```python
from build123d import *

# Parameters (mm, degrees)
F0_W      = 72
F0_H      = 30
F1_DEPTH  = 4
F3_DEPTH  = 5
F4_R      = 3.75
F5_DEPTH  = 9.001
F8_DEPTH  = 15
F10_DEPTH = 25
F12_DEPTH = 3
F13_R     = 1.65
F14_DEPTH = 3


with BuildPart() as f1:
    # F0 (on Top) → F1 (new body)
    with BuildSketch(Plane.XY):
        with BuildLine():
            ThreePointArc((37.445899, 13.116578), (35.981432, 16.652112), (32.445899, 18.116578))
            Line((32.445899, 18.116578), (-32.554101, 18.116578))
            ThreePointArc((-32.554101, 18.116578), (-36.089635, 16.652112), (-37.554101, 13.116578))
            Line((-37.554101, 13.116578), (-37.554101, -9.883422))
            Line((-37.554101, -9.883422), (-37.554101, -14.883422))
            Line((-37.554101, -14.883422), (-32.554101, -14.883422))
            Line((-32.554101, -14.883422), (32.445899, -14.883422))
            ThreePointArc((32.445899, -14.883422), (35.981432, -13.418956), (37.445899, -9.883422))
            Line((37.445899, -9.883422), (37.445899, 13.116578))
        make_face()
        with Locations((-0.054101, 1.616578)):
            Rectangle(F0_W, F0_H, mode=Mode.SUBTRACT)
    extrude(amount=F1_DEPTH)

    # F2 (on face) → F3 (join)
    with BuildSketch(Plane(origin=(0, 0, 0), x_dir=(1, 0, 0), z_dir=(0, 0, -1))):
        with BuildLine():
            Line((32.445899, 14.883422), (-37.554101, 14.883422))
            Line((-37.554101, 14.883422), (-37.554101, -13.116578))
            ThreePointArc((-37.554101, -13.116578), (-36.089635, -16.652112), (-32.554101, -18.116578))
            Line((-32.554101, -18.116578), (32.445899, -18.116578))
            ThreePointArc((32.445899, -18.116578), (35.981432, -16.652112), (37.445899, -13.116578))
            Line((37.445899, -13.116578), (37.445899, 9.883422))
            ThreePointArc((37.445899, 9.883422), (35.981432, 13.418956), (32.445899, 14.883422))
        make_face()
    extrude(amount=F3_DEPTH)

    # F4 (on face) → F5 (cut, through all)
    with BuildSketch(Plane(origin=(0, 0, -5), x_dir=(1, 0, 0), z_dir=(0, 0, -1))):
        with Locations((8, -1.616578)):
            Circle(F4_R)
    extrude(amount=-F5_DEPTH, mode=Mode.SUBTRACT)

    # F7 (on face) → F8 (join)
    with BuildSketch(Plane(origin=(0, 0, -5), x_dir=(1, 0, 0), z_dir=(0, 0, -1))):
        with BuildLine():
            ThreePointArc((2.992242, -13.613343), (-5, -1.616578), (2.992242, 10.380186))
            Line((2.992242, 10.380186), (2.992242, 11.45715))
            ThreePointArc((2.992242, 11.45715), (-6, -1.616578), (2.992242, -14.690306))
            Line((2.992242, -14.690306), (2.992242, -13.613343))
        make_face()
        with BuildLine():
            ThreePointArc((13.007758, -14.690306), (22, -1.616578), (13.007758, 11.45715))
            Line((13.007758, 11.45715), (13.007758, 10.380186))
            ThreePointArc((13.007758, 10.380186), (21, -1.616578), (13.007758, -13.613343))
            Line((13.007758, -13.613343), (13.007758, -14.690306))
        make_face()
    extrude(amount=F8_DEPTH)

    # F9 (on face) → F10 (cut)
    with BuildSketch(Plane.XY):
        with BuildLine():
            ThreePointArc((19, 0.116578), (20.06066, 0.555918), (20.5, 1.616578))
            ThreePointArc((20.5, 1.616578), (20.06066, 2.677238), (19, 3.116578))
            ThreePointArc((19, 3.116578), (17.5, 1.616578), (19, 0.116578))
        make_face()
        with BuildLine():
            ThreePointArc((19, 0.116578), (17.5, 1.616578), (19, 3.116578))
            Line((19, 3.116578), (-3, 3.116578))
            ThreePointArc((-3, 3.116578), (-1.93934, 2.677238), (-1.5, 1.616578))
            ThreePointArc((-1.5, 1.616578), (-1.93934, 0.555918), (-3, 0.116578))
            Line((-3, 0.116578), (19, 0.116578))
        make_face()
        with BuildLine():
            ThreePointArc((-1.5, 1.616578), (-1.93934, 2.677238), (-3, 3.116578))
            ThreePointArc((-3, 3.116578), (-4.5, 1.616578), (-3, 0.116578))
            ThreePointArc((-3, 0.116578), (-1.93934, 0.555918), (-1.5, 1.616578))
        make_face()
    extrude(amount=-F10_DEPTH, mode=Mode.SUBTRACT)

    # F11 (on face) → F12 (cut)
    with BuildSketch(Plane.XY):
        with BuildLine():
            ThreePointArc((-3, -0.883422), (-1.232233, -0.151189), (-0.5, 1.616578))
            ThreePointArc((-0.5, 1.616578), (-1.232233, 3.384345), (-3, 4.116578))
            ThreePointArc((-3, 4.116578), (-5.5, 1.616578), (-3, -0.883422))
        make_face()
        with BuildLine():
            ThreePointArc((-3, 4.116578), (-1.232233, 3.384345), (-0.5, 1.616578))
            ThreePointArc((-0.5, 1.616578), (-1.232233, -0.151189), (-3, -0.883422))
            Line((-3, -0.883422), (19, -0.883422))
            ThreePointArc((19, -0.883422), (16.5, 1.616578), (19, 4.116578))
            Line((19, 4.116578), (-3, 4.116578))
        make_face()
        with BuildLine():
            ThreePointArc((21.5, 1.616578), (20.767767, 3.384345), (19, 4.116578))
            ThreePointArc((19, 4.116578), (16.5, 1.616578), (19, -0.883422))
            ThreePointArc((19, -0.883422), (20.767767, -0.151189), (21.5, 1.616578))
        make_face()
    extrude(amount=-F12_DEPTH, mode=Mode.SUBTRACT)

    # F13 (on face) → F14 (cut)
    with BuildSketch(Plane.XY):
        with Locations((-24, 1.470634)):
            Circle(F13_R)
        with Locations((-8, 1.470634)):
            Circle(F13_R)
        with Locations((8, 1.470634)):
            Circle(F13_R)
        with Locations((24, 1.470634)):
            Circle(F13_R)
    extrude(amount=-F14_DEPTH, mode=Mode.SUBTRACT)


solid = f1.part
```
The model under review builds one solid part; all positions refer to its coordinate system, in mm. A direction names the side the tool comes from. Give positions to 0.01 mm unless a question says otherwise; leave off trailing zeros. Write each loop counter-clockwise with the first axis right and the second up, starting at its lowest first coordinate (ties: lowest second). Pieces come first, ordered by that corner, then holes. Notation, with made-up numbers: M -19.75,1 L 6.25,1 A20 cw 6.25,5 Z; hole C 79,-39 d5. An arc over 180 degrees is marked long. Write each question's results on one line, items separated by ' | '. Start each with the question number.
1. Mouldability with a two-part tool opening along Y and no side actions: class faces 1 (the cylindrical face through (22.35, 1.54, -1.48)), 2 (the flat face through (-11, -14, 4)), 3 (the cylindrical face through (-36.13, 16.61, -0.44)) as released by +Y, released by -Y, zero draft, split by the parting line, or undercut.
2. We need section D-D (y = -6.5). Write out the cut boundary in (x, z), and give its area (3 significant figures).
3. We need section B-B (x = 24). Write out the cut boundary in (y, z).
4. Insertion check: pin 1 Ø8 at (x, y) = (10, -3.5) entering from +Z; pin 2 Ø1.5 at (x, z) = (19, -7) entering from +Y; pin 3 Ø2.5 at (x, y) = (14.5, 2.5) entering from +Z. Each pin has a flat end and moves straight along its axis. Give the tip position at first contact, or say it passes through.
5. We need section A-A (z = -14). Write out the cut boundary in (x, y), and give its area (3 significant figures).
6. We need section C-C (x = 7.5). Write out the cut boundary in (y, z).
7. For faces 4 (the cylindrical face through (-5, 1.8, -12.4)), 5 (the cylindrical face through (7.939, 5.366, -2.535)), 6 (the flat face through (1, -0.883, -1)), list the 3-axis set-ups (+Z, -Z, +X, -X, +Y, -Y) from which the entire face can be reached by the end or side of a thin tool; tool diameter is ignored.
8. For probe 1 along Y at (x, z) = (-24, -2); probe 2 along X at (y, z) = (1, -10.25); probe 3 along X at (y, z) = (5, 2), list the stretches that pass through material, from the lowest coordinate up. Write a range as [from, to].
Results found:
1) face 1: undercut | face 2: zero draft | face 3: released by +Y
2) outline: M -37.55,-5 L -3.41,-5 L -3.41,-20 L -2.15,-20 L -2.15,-5 L 18.15,-5 L 18.15,-20 L 19.41,-20 L 19.41,-5 L 37.45,-5 L 37.45,4 L 35.95,4 L 35.95,0 L -36.05,0 L -36.05,4 L -37.55,4 Z | area: 425 mm^2
3) outline: M -14.88,-5 L 18.12,-5 L 18.12,4 L 16.62,4 L 16.62,0 L 3.12,0 L 3.12,-3 L -0.18,-3 L -0.18,0 L -13.38,0 L -13.38,4 L -14.88,4 Z
4) pin 1: stops at z = 0 | pin 2: stops at y = 11.15 | pin 3: stops at z = -3
5) outline: M 2.99,-11.46 L 2.99,-10.38 A13 cw 2.99,13.61 L 2.99,14.69 A14 ccw Z; M 13.01,-11.46 A14 ccw 13.01,14.69 L 13.01,13.61 A13 cw 13.01,-10.38 Z | area: 64.3 mm^2
6) outline: M -14.88,-5 L -2.1,-5 L -2.1,0 L -13.38,0 L -13.38,4 L -14.88,4 Z; M 5.33,-5 L 18.12,-5 L 18.12,4 L 16.62,4 L 16.62,0 L 5.33,0 Z
7) face 4: -Z | face 5: +Z, -Z | face 6: +Z
8) probe 1: y = [-14.88, -0.18], [3.12, 18.12] | probe 2: x = [-5.99, -4.99], [20.99, 21.99] | probe 3: x = [-37.55, -36.05], [35.95, 37.45]
